The model under review builds one solid part; all positions refer to its coordinate system, in mm. A direction names the side the tool comes from. Round coordinates to 2 decimals unless told otherwise and drop trailing zeros.
Item 1: Machinability: for faces 1 (the face through (8.586, -0.867, -3.905)), 2 (the face through (1.972, -2.627, -1.545)), 3 (the face through (0, -2.5, -2.5)), which of the approach directions +Z, -Z, +X, -X, +Y, -Y give a long, thin tool a straight path to every point of the face, cutting with its end or side? Answer none if there is none.
Item 2: To check wall thickness, follow L1, parallel to Z at x = 5.25, y = -0.25; L2, parallel to X at y = 2.75, z = -5; L3, parallel to X at y = 4.25, z = -4.5. State the ranges of each line that lie inside material, in increasing order.
Item 3: Clearance check with flat-ended pins moving along their axes: pin 1 Ø1.5 at (x, z) = (15, -4) entering from -Y; pin 2 Ø0.8 at (y, z) = (-0.5, 2) entering from -X; pin 3 Ø2 at (x, z) = (12, 4.5) entering from +Y. State where each tip first meets the part, or that it passes through.
```python
from build123d import *

# Parameters (mm, degrees)
FILLET1_R       = 0.4
HEX_2_DEPTH     = 4
THDSCHPAT_COUNT = 15
THDSCHPAT_PITCH = 1.25


with BuildPart() as part:
    # BodySke → Base-Revolve (revolve)
    with BuildSketch(Plane.XY):
        Polygon((0, 0), (0, 5.7), (0.8, 6.5), (8, 6.5), (8, 4), (27.3095, 4), (28, 3.3095), (28, 0), align=None)
    revolve(axis=Axis((-31.75, 0, 0), (1, 0, 0)))

    # Fillet1
    fillet1_edges = [part.edges().sort_by_distance(p)[0] for p in [
        (8, -4, 0),
    ]]
    fillet(fillet1_edges, radius=FILLET1_R)

    # Sketch2 → Hex-PreBroach (revolve, cut)
    with BuildSketch(Plane.XY):
        Polygon((0, 3.0475), (4, 3.0475), (5.759474945, 0), (0, 0), align=None)
    revolve(axis=Axis((0, 0, 0), (1, 0, 0)), mode=Mode.SUBTRACT)

    # Sketch3 → Hex 2 (cut)
    with BuildSketch(Plane(origin=(0, 0, 0), x_dir=(0, 0.5, 0.866025404), z_dir=(-1, 0, 0))):
        Polygon((1.759474945, 3.0475), (-1.759474945, 3.0475), (-3.518949891, 0), (-1.759474945, -3.0475), (1.759474945, -3.0475), (3.518949891, 0), align=None)
    extrude(amount=-HEX_2_DEPTH, mode=Mode.SUBTRACT)

    # ThdSchSke → ThreadSchematic (revolve, cut)
    with BuildSketch(Plane.XY):
        Polygon((9.25, -3.3095), (8.766506695, -4), (8.766506695, -5), (9.733493305, -5), (9.733493305, -4), align=None)
    threadschematic = revolve(axis=Axis((-3.175, 0, 0), (1, 0, 0)), mode=Mode.SUBTRACT)

    # ThdSchPat: ThreadSchematic ×15
    with Locations(*[(i * THDSCHPAT_PITCH, 0, 0) for i in range(1, THDSCHPAT_COUNT)]):
        add(threadschematic, mode=Mode.SUBTRACT)


solid = part.part
```
Numbers:
1. face 1: +X
1. face 2: -X
1. face 3: +Z, -Z, -X, +Y, -Y
2. L1: z = -6.5 to -0.85, 0.85 to 6.5
2. L2: x = 0.01 to 8
2. L3: x = 0.49 to 8
3. pin 1: stops at y = -2.33
3. pin 2: stops at x = 4.34
3. pin 3: stops at y = 1.89
